from build123d import *

# Parameters (mm, degrees)
SKETCH1_R           = 1.25
BOSS_EXTRUDE1_DEPTH = 8.3


with BuildPart() as part:
    # Sketch1 → Boss-Extrude1 (new body)
    with BuildSketch(Plane(origin=(0, 0, 0), x_dir=(1, 0, 0), z_dir=(0, 1, 0))):
        with BuildLine():
            Line((35.434172296, 1.287491613), (35.622727971, 1.3307936))
            ThreePointArc((35.622727971, 1.3307936), (36.223294794, 7.531563888), (32.32905872, 2.668935167))
            ThreePointArc((32.32905872, 2.668935167), (0.027157554, -0.697665471), (-32.309217612, 2.319893124))
            ThreePointArc((-32.309217612, 2.319893124), (-36.261610619, 7.13771657), (-35.575715837, 0.943979283))
            Line((-35.575715837, 0.943979283), (-35.413230424, 0.907951956))
            ThreePointArc((-35.413230424, 0.907951956), (0.030803418, -2.69767479), (35.434172296, 1.287491613))
        make_face()
        with Locations((-35, 4.142580739)):
            Circle(SKETCH1_R, mode=Mode.SUBTRACT)
        with Locations((35, 4.520575704)):
            Circle(SKETCH1_R, mode=Mode.SUBTRACT)
    extrude(amount=BOSS_EXTRUDE1_DEPTH)


solid = part.part
Could you check a few things on this model? Use its own coordinates, in mm. Round coordinates to 2 decimals unless told otherwise and drop trailing zeros. Order: outer loops, then holes, each group sorted by start corner. A loop starts at its lowest first (then second) coordinate and runs counter-clockwise, first axis right, second up.
(1) If we mould it in two halves opening along X, with no side actions, what happens to faces 1 (the flat face through (0, 8.3, 1)), 2 (the cylindrical face through (-0.5, 4.1, 2.7)), 3 (the cylindrical face through (34.01, 4.09, -3.76)), 4 (the cylindrical face through (-35.92, 4.09, -4.99))? For each: released by +X, released by -X, zero draft, split by the parting line, or undercut.
Response values:
face 1: zero draft
face 2: split by the parting line
face 3: undercut
face 4: undercut
(2) Imagine slicing it at D-D (x = 26.5). Write out the boundary of the cut face in (y, z), plus the area to 3 significant figures.
Response values:
outline: (0, -1.58) - (8.3, -1.58) - (8.3, 0.45) - (0, 0.45) - close
area: 16.8 mm2
(3) I'm going to push flat-ended pins straight in: pin 1 (2 mm diameter, centred on y = 3.5, z = -1, fed in from +X); pin 2 (1.5 mm diameter, centred on y = 1.5, z = -3, fed in from -X); pin 3 (2 mm diameter, centred on x = -35, z = -4.14, fed in from +Y). Where does each tip first touch, or does it pass through?
Response values:
pin 1: stops at x = 37.05
pin 2: stops at x = -38.23
pin 3: passes through
(4) Imagine slicing it at B-B (y = 5). Write out the boundary of the cut face in (x, z), plus the area to 3 significant figures.
Response values:
outline: (-35.58, -0.94) arc R3.25 ccw (long way) to (-32.31, -2.32) arc R165.21 cw to (32.33, -2.67) arc R3.25 ccw (long way) to (35.62, -1.33) - (35.43, -1.29) arc R167.21 ccw to (-35.41, -0.91) - close; hole circle Ø2.5 at (-35, -4.14); hole circle Ø2.5 at (35, -4.52)
area: 191 mm2
(5) Please list where these lines run through material, in increasing order: line 1 along X through (y, z) = (7.75, -4.25); line 2 along Z through (x, y) = (35, 6); line 3 along Z through (x, y) = (1, 2.75).
Response values:
line 1: x = -38.25 to -36.25, -33.75 to -31.75, 31.76 to 33.78, 36.22 to 38.24
line 2: z = -7.77 to -5.77, -3.27 to -1.19
line 3: z = 0.69 to 2.69
(6) Imagine slicing it at A-A (z = -6.75). Write out the boundary of the cut face in (x, y).
Response values:
outline: (-36.94, 0) - (-33.06, 0) - (-33.06, 8.3) - (-36.94, 8.3) - close; (32.64, 0) - (37.36, 0) - (37.36, 8.3) - (32.64, 8.3) - close
(7) Imagine slicing it at C-C (x = 4). Write out the boundary of the cut face in (y, z), plus the area to 3 significant figures.
Response values:
outline: (0, 0.63) - (8.3, 0.63) - (8.3, 2.63) - (0, 2.63) - close
area: 16.6 mm2
